Work out the finished part from the listing and answer in its coordinate system (mm). Give positions to 0.01 mm unless a question says otherwise; leave off trailing zeros. Write each loop counter-clockwise with the first axis right and the second up, starting at its lowest first coordinate (ties: lowest second). Pieces come first, ordered by that corner, then holes. Notation, with made-up numbers: (-32.75, 10) - (24.25, 10) arc R23 ccw to (24.25, 18) - close; hole circle Ø1 at (-33, 60.25). An arc over 180 degrees is marked (long way). Write each question's results on one line, items separated by ' | '. Start each with the question number.
from build123d import *

# Parameters (mm, degrees)
BOSS_EXTRUDE1_DEPTH = 0.5588
SKETCH2_R           = 16.9164
SKETCH2_R_2         = 12.7
CUT_EXTRUDE1_DEPTH  = 137.784327529


with BuildPart() as part:
    # Sketch1 → Boss-Extrude1 (new body)
    with BuildSketch(Plane.XY):
        with BuildLine():
            Line((0, 0), (0, 101.6))
            ThreePointArc((0, 101.6), (25.4, 127), (50.8, 101.6))
            Line((50.8, 101.6), (50.8, 0))
            ThreePointArc((50.8, 0), (25.4, -25.4), (0, 0))
        make_face()
    extrude(amount=BOSS_EXTRUDE1_DEPTH)

    # Sketch2 → Cut-Extrude1 (cut, through all)
    with BuildSketch(Plane.XY.offset(0.5588)):
        with Locations((25.4, 101.6)):
            Circle(SKETCH2_R)
        with Locations((25.4, 0)):
            Circle(SKETCH2_R_2)
    extrude(amount=-CUT_EXTRUDE1_DEPTH, mode=Mode.SUBTRACT)


solid = part.part
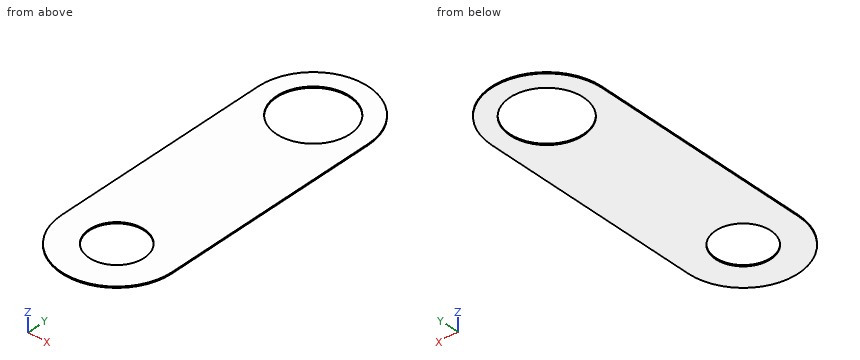
Q1. A cutting plane is placed at C-C, the plane z = 0.1. Write down the section's boundary in (x, y), and give its area (3 significant figures).
Q2. A cutting plane is placed at A-A, the plane x = 25.4. Write down the section's boundary in (y, z), and give its area (3 significant figures).
Q3. A cutting plane is placed at B-B, the plane y = 99. Write down the section's boundary in (x, z).
Q4. Consider L1, parallel to Y at x = 25.4, z = 0.4; L2, parallel to X at y = 8, z = 0.2; L3, parallel to X at y = 114.5, z = 0.3. Determine where each line is inside the solid, lowest interval first.
Q5. A cutting plane is placed at D-D, the plane y = 9.5. Write down the section's boundary in (x, z), and give its area (3 significant figures).
Result:
1) outline: (0, 0) arc R25.4 ccw to (50.8, 0) - (50.8, 101.6) arc R25.4 ccw to (0, 101.6) - close; hole circle Ø33.83 at (25.4, 101.6); hole circle Ø25.4 at (25.4, 0) | area: 5,780 mm2
2) outline: (-25.4, 0) - (-12.7, 0) - (-12.7, 0.56) - (-25.4, 0.56) - close; (12.7, 0) - (84.68, 0) - (84.68, 0.56) - (12.7, 0.56) - close; (118.52, 0) - (127, 0) - (127, 0.56) - (118.52, 0.56) - close | area: 52.1 mm2
3) outline: (0, 0) - (8.68, 0) - (8.68, 0.56) - (0, 0.56) - close; (42.12, 0) - (50.8, 0) - (50.8, 0.56) - (42.12, 0.56) - close
4) L1: y = -25.4 to -12.7, 12.7 to 84.68, 118.52 to 127 | L2: x = 0 to 15.54, 35.26 to 50.8 | L3: x = 3.52 to 14.46, 36.34 to 47.28
5) outline: (0, 0) - (16.97, 0) - (16.97, 0.56) - (0, 0.56) - close; (33.83, 0) - (50.8, 0) - (50.8, 0.56) - (33.83, 0.56) - close | area: 19.0 mm2
